Verification items for the finished model (mm, model axes). Give positions to 0.01 mm unless a question says otherwise; leave off trailing zeros. Write each loop counter-clockwise with the first axis right and the second up, starting at its lowest first coordinate (ties: lowest second). Pieces come first, ordered by that corner, then holes. Notation, with made-up numbers: M -16,75 L -8,75 A29 cw -8,110 Z; hole C 65.5,68.5 d7. An arc over 180 degrees is marked long. Answer as a JSON object with one key per item and string values.
```python
from build123d import *

# Parameters (mm, degrees)
SKETCH1_R             = 6.25
SKETCH1_R_2           = 3.75
SKETCH1_R_3           = 2.5
BOSS_EXTRUDE1_DEPTH   = 5
F_6_CLEARANCE_HOLE1_D = 3.7973


with BuildPart() as part:
    # Sketch1 → Boss-Extrude1 (new body)
    # profile 1 of 15: a face of its own
    with BuildSketch(Plane(origin=(0, 0, 0), x_dir=(1, 0, 0), z_dir=(0, 1, 0))):
        Circle(SKETCH1_R)
    # profile 2 of 15: a face of its own
    with BuildSketch(Plane(origin=(0, 0, 0), x_dir=(1, 0, 0), z_dir=(0, 1, 0))):
        with Locations((-7.75, 0)):
            Circle(SKETCH1_R_2)
        with Locations((-7.75, 0)):
            Circle(SKETCH1_R_3, mode=Mode.SUBTRACT)
    # profile 3 of 15: a face of its own
    with BuildSketch(Plane(origin=(0, 0, 0), x_dir=(1, 0, 0), z_dir=(0, 1, 0))):
        Circle(SKETCH1_R)
    # profile 4 of 15: a face of its own
    with BuildSketch(Plane(origin=(0, 0, 0), x_dir=(1, 0, 0), z_dir=(0, 1, 0))):
        with Locations((-7.75, 0)):
            Circle(SKETCH1_R_2)
        with Locations((-7.75, 0)):
            Circle(SKETCH1_R_3, mode=Mode.SUBTRACT)
    # profile 5 of 15: a face of its own
    with BuildSketch(Plane(origin=(0, 0, 0), x_dir=(1, 0, 0), z_dir=(0, 1, 0))):
        with Locations((7.75, 0)):
            Circle(SKETCH1_R_2)
    # profile 6 of 15: a face of its own
    with BuildSketch(Plane(origin=(0, 0, 0), x_dir=(1, 0, 0), z_dir=(0, 1, 0))):
        Circle(SKETCH1_R)
    # profile 7 of 15: a face of its own
    with BuildSketch(Plane(origin=(0, 0, 0), x_dir=(1, 0, 0), z_dir=(0, 1, 0))):
        with Locations((-7.75, 0)):
            Circle(SKETCH1_R_2)
    # profile 8 of 15: a face of its own
    with BuildSketch(Plane(origin=(0, 0, 0), x_dir=(1, 0, 0), z_dir=(0, 1, 0))):
        with BuildLine():
            ThreePointArc((-5.487903226, -2.990889196), (-7.15425073, -3.702375293), (-8.959677419, -3.54953244))
            Line((-8.959677419, -3.54953244), (-2.016129032, -5.9158874))
            ThreePointArc((-2.016129032, -5.9158874), (-4.026975125, -4.77974595), (-5.487903226, -2.990889196))
        make_face()
    # profile 9 of 15: a face of its own
    with BuildSketch(Plane(origin=(0, 0, 0), x_dir=(1, 0, 0), z_dir=(0, 1, 0))):
        with BuildLine():
            ThreePointArc((5.487903226, -2.990889196), (4.026975125, -4.77974595), (2.016129032, -5.9158874))
            Line((2.016129032, -5.9158874), (8.959677419, -3.54953244))
            ThreePointArc((8.959677419, -3.54953244), (7.15425073, -3.702375293), (5.487903226, -2.990889196))
        make_face()
    # profile 10 of 15: a face of its own
    with BuildSketch(Plane(origin=(0, 0, 0), x_dir=(1, 0, 0), z_dir=(0, 1, 0))):
        Circle(SKETCH1_R)
    # profile 11 of 15: a face of its own
    with BuildSketch(Plane(origin=(0, 0, 0), x_dir=(1, 0, 0), z_dir=(0, 1, 0))):
        with Locations((7.75, 0)):
            Circle(SKETCH1_R_2)
        with Locations((7.75, 0)):
            Circle(SKETCH1_R_3, mode=Mode.SUBTRACT)
    # profile 12 of 15: a face of its own
    with BuildSketch(Plane(origin=(0, 0, 0), x_dir=(1, 0, 0), z_dir=(0, 1, 0))):
        with Locations((7.75, 0)):
            Circle(SKETCH1_R_2)
        with Locations((7.75, 0)):
            Circle(SKETCH1_R_3, mode=Mode.SUBTRACT)
    # profile 13 of 15: a face of its own
    with BuildSketch(Plane(origin=(0, 0, 0), x_dir=(1, 0, 0), z_dir=(0, 1, 0))):
        Circle(SKETCH1_R)
    # profile 14 of 15: a face of its own
    with BuildSketch(Plane(origin=(0, 0, 0), x_dir=(1, 0, 0), z_dir=(0, 1, 0))):
        with BuildLine():
            Line((8.959677419, 3.54953244), (2.016129032, 5.9158874))
            ThreePointArc((2.016129032, 5.9158874), (4.026975125, 4.77974595), (5.487903226, 2.990889196))
            ThreePointArc((5.487903226, 2.990889196), (7.15425073, 3.702375293), (8.959677419, 3.54953244))
        make_face()
    # profile 15 of 15: a face of its own
    with BuildSketch(Plane(origin=(0, 0, 0), x_dir=(1, 0, 0), z_dir=(0, 1, 0))):
        with BuildLine():
            Line((-2.016129032, 5.9158874), (-8.959677419, 3.54953244))
            ThreePointArc((-8.959677419, 3.54953244), (-7.15425073, 3.702375293), (-5.487903226, 2.990889196))
            ThreePointArc((-5.487903226, 2.990889196), (-4.026975125, 4.77974595), (-2.016129032, 5.9158874))
        make_face()
    extrude(amount=BOSS_EXTRUDE1_DEPTH)

    # #6 Clearance Hole1 (through all)
    with Locations(Plane(origin=(0, 5, 0), x_dir=(1, 0, 0), z_dir=(0, 1, 0))):
        with Locations((7.75, 0), (0, 0)):
            Hole(F_6_CLEARANCE_HOLE1_D / 2)


solid = part.part
```
1) Thickness scan on L1, parallel to X at y = 2.15, z = -1.5; L2, parallel to Z at x = 7.75, y = 1.15; L3, parallel to Z at x = 1.5, y = 4.1. Record the ranges inside material, lowest first.
Completed:
{"L1": "x = -11.19 to -1.16, 1.16 to 6.59, 8.91 to 11.19", "L2": "z = -3.96 to -1.9, 1.9 to 3.96", "L3": "z = -6.07 to -1.16, 1.16 to 6.07"}
2) Section check C-C on x = 0. Record the boundary of the cut face in (y, z), and give its area (3 significant figures).
Completed:
{"outline": "M 0,-6.25 L 5,-6.25 L 5,-1.9 L 0,-1.9 Z; M 0,1.9 L 5,1.9 L 5,6.25 L 0,6.25 Z", "area": "43.5 mm2"}
3) Release check for a two-part mould opening along X. For faces 1 (the face through (-1.8, 2.5, -0.6)), 2 (the face through (-5.537, 2.465, 4.716)), 3 (the face through (5.537, 2.465, -4.716)), 4 (the face through (9.647, 2.465, -0.083)) record: pulls with the +X half, pulls with the -X half, needs draft (parallel to the pull), parting line crosses it, or undercut.
Completed:
{"face 1": "undercut", "face 2": "pulls with the -X half", "face 3": "pulls with the +X half", "face 4": "undercut"}
4) Go/stop test with a flat-tipped pin: pin 1 (3 mm diameter, centred on x = 7.75, z = 0, fed in from +Y) (3 decimals). Record where the tip stops, or that it passes through.
Completed:
{"pin 1": "passes through"}
5) Section check A-A on z = 0. Record the boundary of the cut face in (x, y).
Completed:
{"outline": "M -11.5,0 L -1.9,0 L -1.9,5 L -11.5,5 Z; M 1.9,0 L 5.85,0 L 5.85,5 L 1.9,5 Z; M 9.65,0 L 11.5,0 L 11.5,5 L 9.65,5 Z"}
6) Section check D-D on x = 7.75. Record the boundary of the cut face in (y, z), and give its area (3 significant figures).
Completed:
{"outline": "M 0,-3.96 L 5,-3.96 L 5,-1.9 L 0,-1.9 Z; M 0,1.9 L 5,1.9 L 5,3.96 L 0,3.96 Z", "area": "20.6 mm2"}
7) Section check B-B on y = 0.6. Record the boundary of the cut face in (x, z).
Completed:
{"outline": "M -8.96,-3.55 L -2.02,-5.92 A6.25 ccw 2.02,-5.92 L 8.96,-3.55 A3.75 ccw 8.96,3.55 L 2.02,5.92 A6.25 ccw -2.02,5.92 L -8.96,3.55 A3.75 ccw Z; hole C 0,0 d3.8; hole C 7.75,0 d3.8"}
